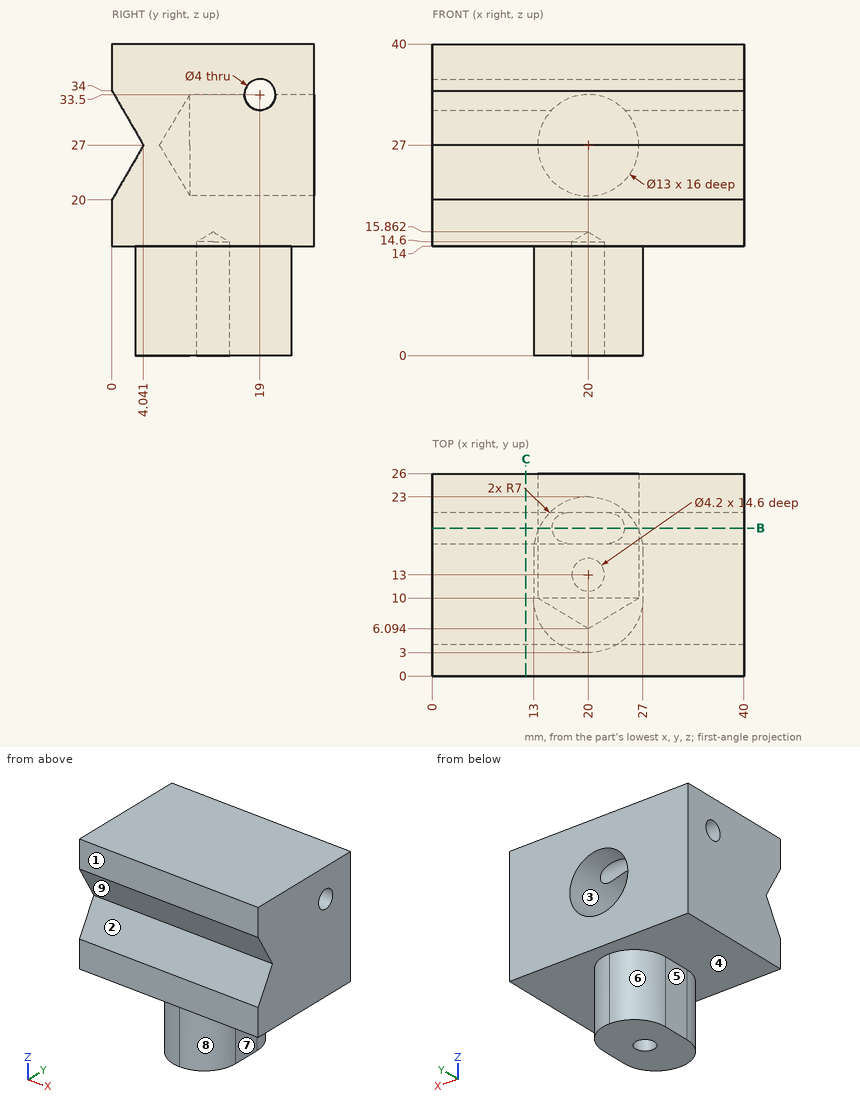
Answer from the drawing. Dimensions are ordinates in mm from the lowest x, y and z of the part. A direction names the side the tool comes from. Round coordinates to 2 decimals unless told otherwise and drop trailing zeros. Loops run counter-clockwise (first coordinate to the right, second up) from the corner with the lowest first, then second, coordinate; pieces in that order, holes last. Notation, with made-up numbers: (77, -33) - (97, -33) arc R29 cw to (97, -5) - close; hole circle Ø7 at (-37, 84). An arc over 180 degrees is marked (long way). Return JSON: item names as keys, results as strings. Group by question number.
1. Each of these flat-tipped pins is pushed along its axis until it touches: P1, Ø5, axis at x = 4.5, y = 14.5, coming from the -Z side; P2, Ø6.5, axis at y = 13.5, z = 6, coming from the +X side; P3, Ø6.5, axis at y = 11.5, z = 9, coming from the -X side. Where does it stop, or does it pass through?
2. The part is cut by section C-C on x = 12. Determine the outline of the cut face in (y, z), then the cut area to 3 significant figures.
3. Consider probe 1 along Y at (x, z) = (20, 11); probe 2 along Z at (x, y) = (28, 19); probe 3 along X at (y, z) = (14, 27). Determine where each line is inside the solid, lowest interval first.
4. Which of the six approach directions +Z, -Z, +X, -X, +Y, -Y give full straight-line access (tool end or side, diameter ignored) to the marked faces 5, 6, 7, 8 and 9?
5. The mould has two halves that part along Z. Classify the marked faces 1, 2, 3 and 4: pulls with the +Z half, pulls with the -Z half, needs draft (parallel to the pull), parting line crosses it, or undercut.
6. The part is cut by section B-B on y = 19. Determine the outline of the cut face in (x, z) (1 decimal).
Resolved:
{
 "1": {"P1": "stops at z = 14", "P2": "stops at x = 27", "P3": "stops at x = 13"},
 "2": {"outline": "(0, 14) - (26, 14) - (26, 40) - (0, 40) - (0, 34) - (4.04, 27) - (0, 20) - close; hole circle Ø4 at (19, 33.5)", "area": "635 mm²"},
 "3": {"probe 1": "y = 3 to 10.9, 15.1 to 23", "probe 2": "z = 14 to 31.5, 35.5 to 40", "probe 3": "x = 0 to 13.5, 26.5 to 40"},
 "4": {"face 5": "-Z, -X, +Y, -Y", "face 6": "-Z, -X, +Y", "face 7": "-Z, +X, +Y, -Y", "face 8": "-Z, +X, -Y", "face 9": "+X, -X, -Y"},
 "5": {"face 1": "needs draft", "face 2": "undercut", "face 3": "undercut", "face 4": "pulls with the -Z half"},
 "6": {"outline": "(0, 14) - (13.7, 14) - (13.7, 0) - (26.3, 0) - (26.3, 14) - (40, 14) - (40, 31.5) - (24.7, 31.5) arc R6.5 cw (long way) to (15.3, 31.5) - (0, 31.5) - close; (0, 35.5) - (40, 35.5) - (40, 40) - (0, 40) - close"}
}
